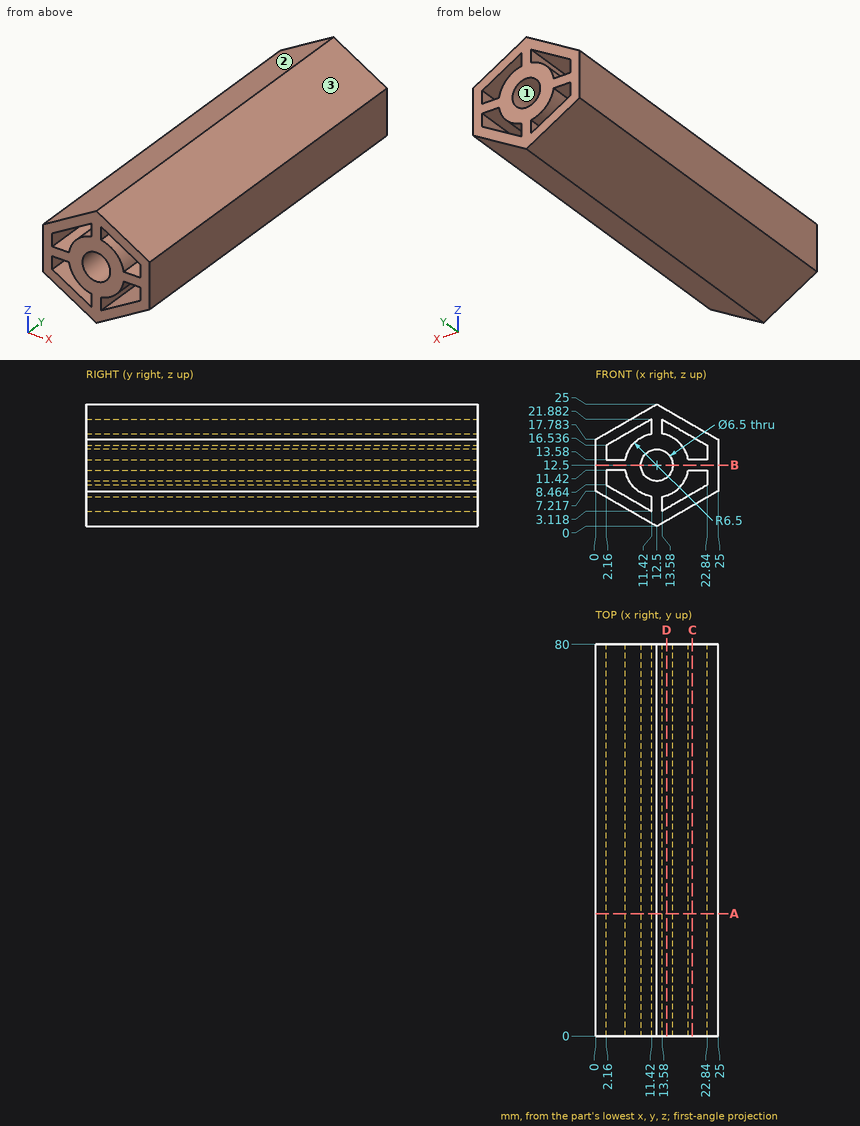
Check sheet for the drawn part. Datum: minimum x, y, z corner. Units: mm. Give positions to 0.01 mm unless a question says otherwise; leave off trailing zeros. Loops run counter-clockwise (first coordinate to the right, second up) from the corner with the lowest first, then second, coordinate; pieces in that order, holes last. Notation, with made-up numbers: (-27.75, -23) - (-9.75, -23) arc R24 cw to (-9.75, -3) - close; hole circle Ø6 at (16, 42). An arc over 180 degrees is marked (long way). Write each question's results on one line, items separated by ' | '.
1) Sectioned sample at A-A on y = 25. Record the boundary of the cut face in (x, z).
Solution:
outline: (0, 7.22) - (12.5, 0) - (25, 7.22) - (25, 17.78) - (12.5, 25) - (0, 17.78) - close; hole (2.16, 8.46) - (11.42, 3.12) - (11.42, 6.09) arc R6.5 cw to (6.09, 11.42) - (2.16, 11.42) - close; hole (2.16, 13.58) - (6.09, 13.58) arc R6.5 cw to (11.42, 18.91) - (11.42, 21.88) - (2.16, 16.54) - close; hole circle Ø6.5 at (12.5, 12.5); hole (13.58, 3.12) - (22.84, 8.46) - (22.84, 11.42) - (18.91, 11.42) arc R6.5 cw to (13.58, 6.09) - close; hole (13.58, 18.91) arc R6.5 cw to (18.91, 13.58) - (22.84, 13.58) - (22.84, 16.54) - (13.58, 21.88) - close
2) Sectioned sample at C-C on x = 19.75. Record the boundary of the cut face in (y, z), plus the area to 3 significant figures.
Solution:
outline: (0, 4.19) - (80, 4.19) - (80, 6.68) - (0, 6.68) - close; (0, 11.42) - (80, 11.42) - (80, 13.58) - (0, 13.58) - close; (0, 18.32) - (80, 18.32) - (80, 20.81) - (0, 20.81) - close | area: 572 mm2
3) Material ranges on L1, parallel to Z at x = 21.5, y = 42.5 (1 decimal); L2, parallel to X at y = 4.5, z = 3.5; L3, parallel to X at y = 70.5, z = 9.75, recorded low to high. Write a range as from..to.
Solution:
L1: 5.2..7.7, 11.4..13.6, 17.3..19.8 | L2: 6.44..10.76, 11.42..13.58, 14.24..18.56 | L3: 0..2.16, 6.61..10.77, 14.23..18.39, 22.84..25
4) Depth check by flat-ended pin: P1, Ø1.5, axis at y = 41, z = 20, coming from the -X side; P2, Ø2, axis at x = 3.5, y = 24.5, coming from the +Z side; P3, Ø2, axis at x = 21.5, y = 58.5, coming from the -Z side. Enter the tip coordinate at first touch or a pass-through.
Solution:
P1: x = 2.54 | P2: z = 20.38 | P3: z = 4.62
5) Sectioned sample at B-B on z = 12.5. Record the boundary of the cut face in (x, y), plus the area to 3 significant figures.
Solution:
outline: (0, 0) - (9.25, 0) - (9.25, 80) - (0, 80) - close; (15.75, 0) - (25, 0) - (25, 80) - (15.75, 80) - close | area: 1,480 mm2
6) Mould release check, pull along X, two halves, no side actions. Record for the marked faces 1, 2 and 3: pulls with the +X half, pulls with the -X half, needs draft (parallel to the pull), parting line crosses it, or undercut.
Solution:
face 1: undercut | face 2: pulls with the -X half | face 3: pulls with the +X half
7) Sectioned sample at D-D on x = 14.5. Record the boundary of the cut face in (y, z) (1 decimal).
Solution:
outline: (0, 1.2) - (80, 1.2) - (80, 3.6) - (0, 3.6) - close; (0, 6.3) - (80, 6.3) - (80, 9.9) - (0, 9.9) - close; (0, 15.1) - (80, 15.1) - (80, 18.7) - (0, 18.7) - close; (0, 21.4) - (80, 21.4) - (80, 23.8) - (0, 23.8) - close
